```python
from build123d import *

# Parameters (mm, degrees)
F0_W     = 8
F0_H     = 8
F1_DEPTH = 3
F2_R     = 3
F2_R_2   = 2
F3_DEPTH = 5


with BuildPart() as f1:
    # F0 (on Front) → F1 (new body)
    with BuildSketch(Plane.XZ):
        Rectangle(F0_W, F0_H)
    extrude(amount=F1_DEPTH)

    # F2 (on face) → F3 (join)
    with BuildSketch(Plane.XZ.offset(3)):
        Circle(F2_R)
        Circle(F2_R_2, mode=Mode.SUBTRACT)
    extrude(amount=F3_DEPTH)


solid = f1.part
```
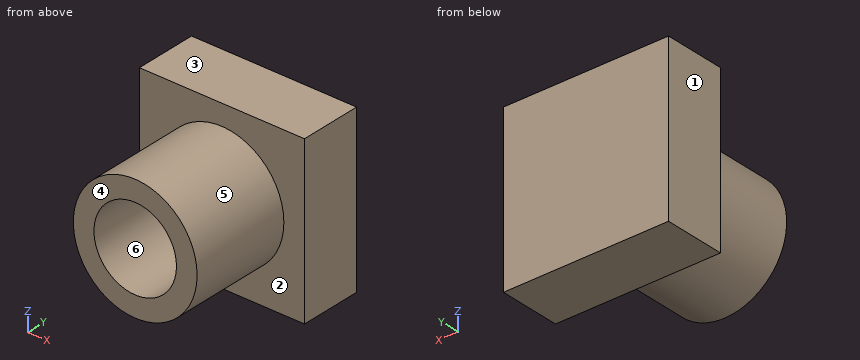
Input: part model. Units: mm. Frame: model coordinates. Face numbers are marked on the shaded views. A direction names the side the tool comes from. Give positions to 0.01 mm unless a question says otherwise; leave off trailing zeros. Loops run counter-clockwise (first coordinate to the right, second up) from the corner with the lowest first, then second, coordinate; pieces in that order, holes last.
1) Line query: L1, parallel to Z at x = 0, y = -4.55; L2, parallel to Y at x = 2.5, z = 3.75; L3, parallel to Z at x = -2.25, y = -7. Output: solid intervals per line, ascending.
A:
L1: z = -3 to -2, 2 to 3
L2: y = -3 to 0
L3: z = -1.98 to 1.98
2) Contact query for flat-ended pins moving along their axis: pin 1 (4 mm diameter, centred on x = 1.5, y = -6.5, fed in from -Z); pin 2 (2 mm diameter, centred on x = 0, z = 0, fed in from -Y); pin 3 (1 mm diameter, centred on y = -4.5, z = -1.5, fed in from -X). Output: stop coordinate, or through.
A:
pin 1: stops at z = -3
pin 2: stops at y = -3
pin 3: stops at x = -2.83
3) Mould query, pull axis Z, two halves, no side actions, for the marked faces 3, 4, 5 and 6. Classes: released by +Z, released by -Z, zero draft, split by the parting line, or undercut.
A:
face 3: released by +Z
face 4: zero draft
face 5: split by the parting line
face 6: undercut
4) Section query C-C on y = -3.5. Return the cut outline in (x, z).
A:
outline: circle Ø6 at (0, 0); hole circle Ø4 at (0, 0)
5) Section query B-B on z = -1.75. Return the cut outline in (x, y).
A:
outline: (-4, -3) - (-2.44, -3) - (-2.44, -8) - (-0.97, -8) - (-0.97, -3) - (0.97, -3) - (0.97, -8) - (2.44, -8) - (2.44, -3) - (4, -3) - (4, 0) - (-4, 0) - close
6) Reachability of the marked faces 1 and 2 from +Z, -Z, +X, -X, +Y, -Y: full face, straight path, thin tool, end or side. Return the list, or none.
A:
face 1: +Z, -Z, -X, +Y, -Y
face 2: -Y
7) Section query A-A on x = 0. Return the cut outline in (y, z).
A:
outline: (-8, -3) - (-3, -3) - (-3, -4) - (0, -4) - (0, 4) - (-3, 4) - (-3, 3) - (-8, 3) - (-8, 2) - (-3, 2) - (-3, -2) - (-8, -2) - close
8) Section query D-D on x = -3.5. Return the cut outline in (y, z).
A:
outline: (-3, -4) - (0, -4) - (0, 4) - (-3, 4) - close
